Input: part model. Units: mm. Frame: model coordinates. A direction names the side the tool comes from. Coordinates: 2 decimals unless noted, no trailing zeros. Order: outer loops, then holes, each group sorted by start corner. A loop starts at its lowest first (then second) coordinate and runs counter-clockwise, first axis right, second up. Notation, with made-up numbers: (7, 63) - (21, 63) arc R14 ccw to (21, 86) - close; hole circle Ø3 at (38, 51.25). An arc over 180 degrees is marked (long way). Answer as CSV lines item,"result". Start each with the question number.
Item 1: Section A-A (x = 242). Output: boundary loops of the cut face in (y, z), and give its area (3 significant figures).
Item 2: Material intervals for line 1 along Y through (x, z) = (250, 0); line 2 along Z through (x, y) = (134, 5); line 3 along X through (y, z) = (-12, 12), sorted ascending.
Item 3: Section B-B (x = 49). Output: boundary loops of the cut face in (y, z), and give its area (3 significant figures).
Item 4: Access query for faces 1 (the cylindrical face through (163.26, 8.43, 4.38)), 2 (the cylindrical face through (19.72, 19.524, -4.336)). Directions: +Z, -Z, +X, -X, +Y, -Y. A direction counts if a zero-diameter tool reaches every point of the face in a straight line with its end or side. Return the directions, or none.
Item 5: First-contact query: pin 1 (2 mm diameter, centred on y = -14.5, z = 2, fed in from +X); pin 2 (12 mm diameter, centred on x = 226, z = 3, fed in from -Y); pin 3 (8 mm diameter, centred on y = -7.5, z = 11, fed in from +X). Flat tips, straight axial feed; report the tip coordinate or a pass-through.
from build123d import *

# Parameters (mm, degrees)
F2_R = 2


with BuildPart() as f1:
    # F0 (on Front) → F1 (revolve)
    with BuildSketch(Plane.XZ):
        with BuildLine():
            Line((0, 0), (267, 0))
            Line((267, 0), (267, 6))
            Line((267, 6), (181, 6))
            Line((181, 6), (181, 9.5))
            Line((181, 9.5), (146, 9.5))
            Line((146, 9.5), (136.669873, 12))
            Line((136.669873, 12), (46.669873, 12))
            ThreePointArc((46.669873, 12), (44.341818, 16.839471), (40, 20))
            Line((40, 20), (0, 20))
            Line((0, 20), (0, 0))
        make_face()
    revolve(axis=Axis((133.5, 0, 0), (1, 0, 0)))

    # F2
    f2_edges = [f1.edges().sort_by_distance(p)[0] for p in [
        (267, 0, -6),
    ]]
    fillet(f2_edges, radius=F2_R)


solid = f1.part
Determined:
1,outline,"circle Ø12 at (0, 0)"
1,area,"113 mm^2"
2,line 1,"y = -6 to 6"
2,line 2,"z = -10.91 to 10.91"
2,line 3,"x = 0 to 44.23"
3,outline,"circle Ø24 at (0, 0)"
3,area,"452 mm^2"
4,face 1,"+X"
4,face 2,"+X, -X"
5,pin 1,"stops at x = 46.2"
5,pin 2,"stops at y = -6"
5,pin 3,"stops at x = 181"
